Autodesk Inventor part; units mm, degrees
ref_plane "YZ Plane" through (0, 0, 0) normal (1, 0, 0) x (0, 1, 0)
ref_plane "XZ Plane" through (0, 0, 0) normal (0, 1, 0) x (-1, 0, 0)
ref_plane "XY Plane" through (0, 0, 0) normal (0, 0, 1) x (1, 0, 0)
sketch "Sketch1" plane through (0, 0, 0) normal (0, 0, 1) x (1, 0, 0)
  circle A0 centre (0, 0) radius 5.5
  dimension "d0" = 11
extrude "Extrusion1" add sketch "Sketch1" along normal blind 10
sketch "Sketch2" plane through (0, 0, 10) normal (0, 0, 1) x (1, 0, 0)
  circle A0 centre (0, 0) radius 11.15
  dimension "d3" = 22.3
extrude "Extrusion3" add sketch "Sketch2" along normal blind 44
sketch "Sketch3" plane through (0, 0, 10) normal (0, 0, -1) x (-1, 0, 0)
  circle A0 centre (0, 0) radius 10.15
  circle A1 centre (0, 0) radius 11.15
  dimension "d8" = 20.3
  dimension "d9" = 22.3
extrude "Extrusion4" add sketch "Sketch3" along normal blind 5
sketch "Sketch4" plane through (0, 0, 54) normal (0, 0, 1) x (1, 0, 0)
  circle A0 centre (0, 0) radius 14.45
  dimension "d12" = 28.9
extrude "Extrusion5" add sketch "Sketch4" along normal blind 20
fillet "Fillet1" radius 2 1 edges at (-14.45, 0, 74)
fillet "Fillet2" radius 2 1 edges at (-5.5, 0, 0)
fillet "Fillet3" radius 2 1 edges at (11.15, 0, 5)
fillet "Fillet4" radius 2 1 edges at (-14.45, 0, 54)
properties part number "Elbow_Parallel_Rod_V1"
For this review, take the finished solid that the model builds, in its own axes (mm). A direction names the side the tool comes from. Round coordinates to 2 decimals unless told otherwise and drop trailing zeros. Order: outer loops, then holes, each group sorted by start corner. A loop starts at its lowest first (then second) coordinate and runs counter-clockwise, first axis right, second up. Notation, with made-up numbers: (-34.5, 0.5) -> (11.5, 0.5) arc R36 cw to (11.5, 37.5) -> close; hole circle Ø10 at (-6, -15). An arc over 180 degrees is marked (long way). Use a Markdown table: item, result.
Item 1: For line 1 along Y through (x, z) = (0, 6.55); line 2 along Y through (x, z) = (0, 6.05); line 3 along Z through (x, y) = (-8.25, -0.5), list the stretches that pass through material, from the lowest coordinate up. Write a range as [from, to].
Resolved:
| item | result |
|---|---|
| line 1 | y = [-11.14, -10.15], [-5.5, 5.5], [10.15, 11.14] |
| line 2 | y = [-11.03, -10.15], [-5.5, 5.5], [10.15, 11.03] |
| line 3 | z = [10, 74] |
Item 2: Take a section at C-C (z = 69.5). State the section outline as (x, y) points, plus the area to 3 significant figures.
Resolved:
| item | result |
|---|---|
| outline | circle Ø28.9 at (0, 0) |
| area | 656 mm² |
Item 3: Take a section at B-B (z = 28.5). State the section outline as (x, y) points.
Resolved:
| item | result |
|---|---|
| outline | circle Ø22.3 at (0, 0) |
Item 4: Take a section at A-A (x = 0). State the section outline as (y, z) points.
Resolved:
| item | result |
|---|---|
| outline | (-14.45, 56) arc R2 ccw to (-12.45, 54) -> (-11.15, 54) -> (-11.15, 6.73) arc R2 ccw to (-10.15, 5) -> (-10.15, 10) -> (-5.5, 10) -> (-5.5, 2) arc R2 ccw to (-3.5, 0) -> (3.5, 0) arc R2 ccw to (5.5, 2) -> (5.5, 10) -> (10.15, 10) -> (10.15, 5) arc R2 ccw to (11.15, 6.73) -> (11.15, 54) -> (12.45, 54) arc R2 ccw to (14.45, 56) -> (14.45, 72) arc R2 ccw to (12.45, 74) -> (-12.45, 74) arc R2 ccw to (-14.45, 72) -> close |
Item 5: Draft analysis for pull direction X (two halves, no side actions). For faces 3 (the flat face through (4, -4, 10)), 4 (the flat face through (0, 0, 0)), 5 (the cylindrical face through (7.768, -12.184, 63.888)), 6 (the cylindrical face through (-1.19, 5.37, 5.94)), state which applies: +X half, -X half, draft (parallel to the pull), parting line (faces both ways), or undercut.
Resolved:
| item | result |
|---|---|
| face 3 | undercut |
| face 4 | draft |
| face 5 | parting line |
| face 6 | undercut |
Item 6: Machinability: for faces 1 (the flat face through (-3, -11, 54)), 2 (the flat face through (0, 0, 74)), which of the approach directions +Z, -Z, +X, -X, +Y, -Y give a long, thin tool a straight path to every point of the face, cutting with its end or side? Answer none if there is none.
Resolved:
| item | result |
|---|---|
| face 1 | -Z |
| face 2 | +Z, +X, -X, +Y, -Y |
Item 7: For pin 1 (1.5 mm diameter, centred on x = -8.5, z = 47.5, fed in from +Y); pin 2 (6 mm diameter, centred on x = 2, y = 0, fed in from -Z); pin 3 (6 mm diameter, centred on x = -6.5, z = 56.5, fed in from -Y); pin 4 (5 mm diameter, centred on x = 8.5, z = 33.5, fed in from -Y), all flat-tipped, find the tip position at first contact; note any pin that passes through.
Resolved:
| item | result |
|---|---|
| pin 1 | stops at y = 8.02 |
| pin 2 | stops at z = 0 |
| pin 3 | stops at y = -14.02 |
| pin 4 | stops at y = -9.4 |
